from build123d import *

# Parameters (mm, degrees)
F0_W     = 102.5
F0_H     = 27
F1_DEPTH = 17
F3_DEPTH = 190
F4_R     = 12.5
F5_DEPTH = 25
F6_W     = 7
F6_H     = 5
F7_DEPTH = 2


with BuildPart() as f1:
    # F0 (on Front) → F1 (new body)
    with BuildSketch(Plane.XZ):
        Rectangle(F0_W, F0_H)
    extrude(amount=F1_DEPTH)

    # F2 (on face) → F3 (cut)
    with BuildSketch(Plane(origin=(0, 0, -13.5), x_dir=(1, 0, 0), z_dir=(0, 0, -1))):
        Polygon((-51.25, 7), (-26.25, 17), (-51.25, 17), align=None)
        Polygon((51.25, 17), (26.25, 17), (51.25, 7), align=None)
    extrude(amount=-F3_DEPTH, mode=Mode.SUBTRACT)

    # F4 (on face) → F5 (cut)
    with BuildSketch(Plane.XZ.offset(17)):
        with Locations((-53.75, 4)):
            Circle(F4_R)
        with Locations((53.75, 4)):
            Circle(F4_R)
    extrude(amount=-F5_DEPTH, mode=Mode.SUBTRACT)

    # F6 (on face) → F7 (cut)
    with BuildSketch(Plane.XY.offset(13.5)):
        with Locations((17.5, -12.5)):
            Rectangle(F6_W, F6_H)
        with Locations((-17.5, -12.5)):
            Rectangle(F6_W, F6_H)
    extrude(amount=-F7_DEPTH, mode=Mode.SUBTRACT)


solid = f1.part
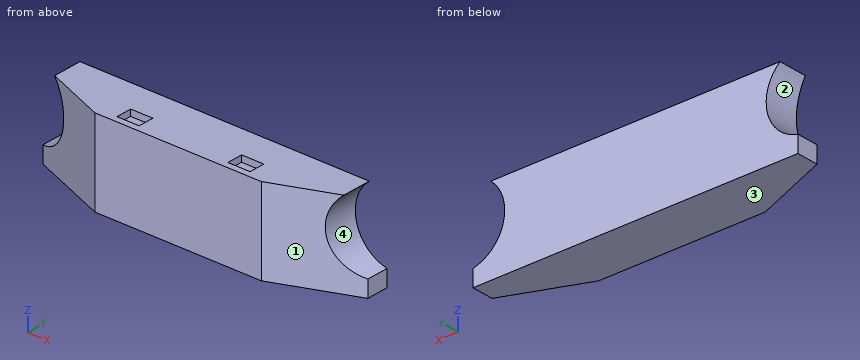
Source: CAD feature listing. Evaluate the final solid. Frame: model axes, mm. Face numbers are marked on the shaded views. Round coordinates to 2 decimals unless told otherwise and drop trailing zeros. Loops run counter-clockwise (first coordinate to the right, second up) from the corner with the lowest first, then second, coordinate; pieces in that order, holes last. Notation, with made-up numbers: (69, 33) - (90, 33) arc R14 ccw to (90, 58) - close; hole circle Ø7 at (-33.5, 17). An arc over 180 degrees is marked (long way). Write item = value, one per line. Start each with the question number.
Item 1: Section query A-A on y = -14. Output: boundary loops of the cut face in (x, z), plus the area to 3 significant figures.
Item 2: First-contact query: pin 1 Ø2.5 at (x, y) = (18, -11.5) entering from +Z; pin 2 Ø8 at (x, z) = (-27, 8.5) entering from -Y; pin 3 Ø3 at (y, z) = (-15, 9.5) entering from -X; pin 4 Ø1.5 at (y, z) = (-10, 10.5) entering from -X. Flat tips, straight axial feed; report the tip coordinate or a pass-through.
Item 3: Mould query, pull axis Z, two halves, no side actions, for the marked faces 1, 2, 3 and 4. Classes: released by +Z, released by -Z, zero draft, split by the parting line, or undercut.
Item 4: Section query B-B on z = 2.75. Output: boundary loops of the cut face in (x, y).
Item 5: Section query C-C on x = -36.5. Output: boundary loops of the cut face in (y, z).
Item 6: Section query D-D on y = -2.25. Output: boundary loops of the cut face in (x, z).
Item 7: Material intervals for line 1 (X direction, y = -2.25, z = 5); line 2 (X direction, y = -8.25, z = -1.25); line 3 (Y direction, x = -31, z = -6), sorted ascending.
Results list:
q1.outline = (-33.75, -13.5) - (33.75, -13.5) - (33.75, 13.5) - (21, 13.5) - (21, 11.5) - (14, 11.5) - (14, 13.5) - (-14, 13.5) - (-14, 11.5) - (-21, 11.5) - (-21, 13.5) - (-33.75, 13.5) - close
q1.area = 1,790 mm²
q2.pin_1 = 11.5
q2.pin_2 = -17
q2.pin_3 = -35
q2.pin_4 = -43.57
q3.face_1 = zero draft
q3.face_2 = undercut
q3.face_3 = released by -Z
q3.face_4 = undercut
q4.outline = (-41.31, -10.97) - (-26.25, -17) - (26.25, -17) - (41.31, -10.97) - (41.31, 0) - (-41.31, 0) - close
q5.outline = (-12.9, -13.5) - (0, -13.5) - (0, 13.5) - (-12.9, 13.5) - close
q6.outline = (-51.25, -13.5) - (51.25, -13.5) - (51.25, -8.25) arc R12.5 cw to (45.63, 13.5) - (-45.63, 13.5) arc R12.5 cw to (-51.25, -8.25) - close
q7.line_1 = -41.29 to 41.29
q7.line_2 = -42.41 to 42.41
q7.line_3 = -15.1 to 0
